Can you work these out from the model? Positions are in its coordinate system, mm. A direction names the side the tool comes from. Coordinates: 2 decimals unless noted, no trailing zeros. Loops run counter-clockwise (first coordinate to the right, second up) from the corner with the lowest first, then second, coordinate; pieces in that order, holes last. Notation, with made-up numbers: M 14,-17 L 67,-17 A25 ccw 67,-1 Z; hole C 38.25,11.25 d7. An arc over 180 degrees is marked long. Answer as a JSON object with one key per item and string values. Group by question number.
Item 1: If I drill on line 1 (Y direction, x = 9.5, z = -12.75); line 2 (X direction, y = 14.5, z = -17), over which ranges is the centre line in solid material (lowest first)?
Item 2: We'd pull the mould along X, two halves only. Please class faces 1 (the flat face through (0, 10, -10)), 2 (the flat face through (6.35, 10, -10)), 3 (the flat face through (13, 17, 0)): +X half, -X half, draft (parallel to the pull), parting line (faces both ways), or undercut.
Item 3: Suppose I cut it at C-C (x = 18.25). Write out the boundary of the cut face in (y, z).
Item 4: Suppose I cut it at A-A (y = 9). Write out the boundary of the cut face in (x, z).
Item 5: Suppose I cut it at B-B (z = -12.5). Write out the boundary of the cut face in (x, y).
Item 6: I'm going to push a flat-ended pin straight in: pin 1 Ø10 at (x, z) = (9, -13) entering from -Y. Where does the tip first touch, or does it pass through?
Item 7: Which directions (+Z, -Z, +X, -X, +Y, -Y) give clear straight access to the entire face, cutting with the end or side of a thin tool? Please do faces 4 (the flat face through (13, 16.51, -10)), 5 (the flat face through (13, 17, -20.638)).
Autodesk Inventor part; units mm, degrees
ref_plane "YZ Plane" through (0, 0, 0) normal (1, 0, 0) x (0, 1, 0)
ref_plane "XZ Plane" through (0, 0, 0) normal (0, 1, 0) x (-1, 0, 0)
ref_plane "XY Plane" through (0, 0, 0) normal (0, 0, 1) x (1, 0, 0)
sketch "Sketch1" plane through (0, 0, 0) normal (0, 0, 1) x (1, 0, 0)
  line L0 (0, 0) -> (25.4, 0)
  line L1 (25.4, 0) -> (25.4, 20.6375)
  line L2 (25.4, 20.6375) -> (0, 20.6375)
  line L3 (0, 20.6375) -> (0, 0)
  line L4 (6.35, 3.81) -> (19.05, 3.81)
  line L5 (19.05, 3.81) -> (19.05, 16.51)
  line L6 (19.05, 16.51) -> (6.35, 16.51)
  line L7 (6.35, 16.51) -> (6.35, 3.81)
  point P0 (0, 10.3188)
  point P1 (12.7, 20.6375)
  dimension "d0" = 25.4
  dimension "d1" = 20.6375
  dimension "d22" = 12.7
  dimension "d23" = 12.7
  dimension "d24" = 6.35
  dimension "d25" = 4.1275
extrude "Extrusion2" add sketch "Sketch1" against normal blind 20.6375
properties part number "Wheel_axle_inner_spacer"
From the geometry:
{
 "1": {"line 1": "0 to 3.81, 16.51 to 20.64", "line 2": "0 to 6.35, 19.05 to 25.4"},
 "2": {"face 1": "-X half", "face 2": "undercut", "face 3": "draft"},
 "3": {"outline": "M 0,-20.64 L 3.81,-20.64 L 3.81,0 L 0,0 Z; M 16.51,-20.64 L 20.64,-20.64 L 20.64,0 L 16.51,0 Z"},
 "4": {"outline": "M 0,-20.64 L 6.35,-20.64 L 6.35,0 L 0,0 Z; M 19.05,-20.64 L 25.4,-20.64 L 25.4,0 L 19.05,0 Z"},
 "5": {"outline": "M 0,0 L 25.4,0 L 25.4,20.64 L 0,20.64 Z; hole M 6.35,3.81 L 19.05,3.81 L 19.05,16.51 L 6.35,16.51 Z"},
 "6": {"pin 1": "y = 0"},
 "7": {"face 4": "+Z, -Z", "face 5": "-Z, +X, -X, +Y, -Y"}
}
